Build history of the part. All positions in model axes, mm. A direction names the side the tool comes from. Give positions to 0.01 mm unless a question says otherwise; leave off trailing zeros. Write each loop counter-clockwise with the first axis right and the second up, starting at its lowest first coordinate (ties: lowest second). Pieces come first, ordered by that corner, then holes. Notation, with made-up numbers: (88.5, -1) -> (117.5, -1) arc R36 cw to (117.5, 38) -> close; hole circle Ø1 at (24.5, 42.25). An arc over 180 degrees is marked (long way). Put each result on its own line as item: value. Start each with the question number.
Item 1: Drill centre lines: line 1 along X through (y, z) = (2.5, 4); line 2 along X through (y, z) = (-0.75, 3.5); line 3 along Y through (x, z) = (-39.5, 2.85). Where is each one in solid material? Low to high.
Item 2: Tool access for faces 5 (the flat face through (58, 1.5, 3)), 6 (the flat face through (-8, 9.1, 3)), 7 (the flat face through (-55, -2.65, 3)), 8 (the flat face through (-51.935, 0, 3)): list every direction of +Z, -Z, +X, -X, +Y, -Y with a clear straight run to the whole face (end or side of a thin tool).
Item 3: Flat gauge pins, fed straight in: pin 1 Ø0.9 at (y, z) = (0.5, 1.5) entering from +X; pin 2 Ø3 at (x, z) = (13.5, 3.5) entering from -Y; pin 3 Ø1.7 at (x, z) = (-34, 2.5) entering from +Y. Where does each tip first touch, or does it go through?
Item 4: Slice it at A-A, the plane x = 2.5. List the corners of the cut face in (y, z), plus the area to 3 significant figures.
Item 5: Two-plate mould, pull along X, no slides. Class faces 1 (the cylindrical face through (60.14, 11.7, 2.83)), 2 (the flat face through (-55, 2.65, 3)), 3 (the flat face through (55, 2.65, 3)), 4 (the flat face through (-59, 1.5, 3)): pulls with the +X half, pulls with the -X half, needs draft (parallel to the pull), parting line crosses it, or undercut.
```python
from build123d import *

# Parameters (mm, degrees)
F1_DEPTH = 5.588
F2_W     = 20
F2_H     = 5.588
F3_DEPTH = 3.5
F4_SIZE2 = 6.99999
F4_SIZE  = 3.49999
F5_W     = 20
F5_H     = 5.588
F6_DEPTH = 3.5
F7_SIZE2 = 3.49999
F7_SIZE  = 6.99999
F8_R     = 3


# Not quite as in the source:
# - a fillet or chamfer is up to 0.001 mm smaller than in the source, because OpenCascade refuses the exact size


with BuildPart() as f1:
    # F0 (on Top) → F1 (new body)
    with BuildSketch(Plane.XY):
        with BuildLine():
            Line((61, 9.1), (-59, 9.1))
            ThreePointArc((-59, 9.1), (-60.4142135624, 8.5142135624), (-61, 7.1))
            Line((-61, 7.1), (-61, 1.5))
            Line((-61, 1.5), (-56, 1.5))
            Line((-56, 1.5), (-56, 2.65))
            Line((-56, 2.65), (-53.7, 2.65))
            Line((-53.7, 2.65), (-53.7, 1.5))
            Line((-53.7, 1.5), (-51.934869796, 1.5))
            Line((-51.934869796, 1.5), (-51.934869796, -1.5))
            Line((-51.934869796, -1.5), (-53.7, -1.5))
            Line((-53.7, -1.5), (-53.7, -2.65))
            Line((-53.7, -2.65), (-56, -2.65))
            Line((-56, -2.65), (-56, -1.5))
            Line((-56, -1.5), (-61, -1.5))
            Line((-61, -1.5), (-61, -7.1))
            ThreePointArc((-61, -7.1), (-60.4142135624, -8.5142135624), (-59, -9.1))
            Line((-59, -9.1), (61, -9.1))
            Line((61, -9.1), (61, -7.1))
            Line((61, -7.1), (61, -1.5))
            Line((61, -1.5), (56, -1.5))
            Line((56, -1.5), (56, -2.65))
            Line((56, -2.65), (53.7, -2.65))
            Line((53.7, -2.65), (53.7, -1.5))
            Line((53.7, -1.5), (51.934869796, -1.5))
            Line((51.934869796, -1.5), (51.934869796, 1.5))
            Line((51.934869796, 1.5), (53.7, 1.5))
            Line((53.7, 1.5), (53.7, 2.65))
            Line((53.7, 2.65), (56, 2.65))
            Line((56, 2.65), (56, 1.5))
            Line((56, 1.5), (61, 1.5))
            Line((61, 1.5), (61, 7.1))
            Line((61, 7.1), (61, 9.1))
        make_face()
    extrude(amount=F1_DEPTH)

    # F2 (on face) → F3 (join)
    with BuildSketch(Plane(origin=(0, 9.1, 0), x_dir=(-1, 0, 0), z_dir=(0, 1, 0))):
        with Locations((-51, 2.794)):
            Rectangle(F2_W, F2_H)
    extrude(amount=F3_DEPTH)

    # F4 (size 3.5 and 7 in the source; OpenCascade refuses exactly that, so slightly less here)
    f4_edges = [f1.edges().sort_by_distance(p)[0] for p in [
        (41, 12.6, 2.794),
    ]]
    f4_side = f1.faces().sort_by_distance((41, 10.85, 2.794))[0]
    chamfer(f4_edges, length=F4_SIZE, length2=F4_SIZE2, reference=f4_side)

    # F5 (on face) → F6 (join)
    with BuildSketch(Plane.XZ.offset(9.1)):
        with Locations((51, 2.794)):
            Rectangle(F5_W, F5_H)
    extrude(amount=F6_DEPTH)

    # F7 (size 7 and 3.5 in the source; OpenCascade refuses exactly that, so slightly less here)
    f7_edges = [f1.edges().sort_by_distance(p)[0] for p in [
        (41, -12.6, 2.794),
    ]]
    f7_side = f1.faces().sort_by_distance((51, -12.6, 2.794))[0]
    chamfer(f7_edges, length=F7_SIZE, length2=F7_SIZE2, reference=f7_side)

    # F8
    f8_edges = [f1.edges().sort_by_distance(p)[0] for p in [
        (61, 12.6, 2.794),
        (61, -12.6, 2.794),
    ]]
    fillet(f8_edges, radius=F8_R)


solid = f1.part
```
Values follow:
1. line 1: -61 to -56, -53.7 to 53.7, 56 to 61
1. line 2: -51.93 to 51.93
1. line 3: -9.1 to 9.1
2. face 5: +Z, -Z, +X
2. face 6: +Z, -Z, -X, +Y
2. face 7: +Z, -Z
2. face 8: +Z, -Z, -X
3. pin 1: x = 51.93
3. pin 2: y = -9.1
3. pin 3: y = 9.1
4. outline: (-9.1, 0) -> (9.1, 0) -> (9.1, 5.59) -> (-9.1, 5.59) -> close
4. area: 102 mm2
5. face 1: pulls with the +X half
5. face 2: undercut
5. face 3: undercut
5. face 4: needs draft
